from build123d import *

# Parameters (mm, degrees)
F0_W     = 50.8
F0_H     = 450.85
F0_R     = 3.770313
F1_DEPTH = 12.7
F2_R     = 4.167188
F3_DEPTH = 25.4
F5_DEPTH = 6.35


with BuildPart() as f1:
    # F0 (on Top) → F1 (new body)
    with BuildSketch(Plane.XY):
        Rectangle(F0_W, F0_H)
        with Locations((-17.5, -215.425)):
            Circle(F0_R, mode=Mode.SUBTRACT)
        with Locations((-17.5, -180.425)):
            Circle(F0_R, mode=Mode.SUBTRACT)
        with Locations((17.5, -215.425)):
            Circle(F0_R, mode=Mode.SUBTRACT)
        with Locations((17.5, -180.425)):
            Circle(F0_R, mode=Mode.SUBTRACT)
        with Locations((-17.5, 180.425)):
            Circle(F0_R, mode=Mode.SUBTRACT)
        with Locations((-17.5, 215.425)):
            Circle(F0_R, mode=Mode.SUBTRACT)
        with Locations((17.5, 180.425)):
            Circle(F0_R, mode=Mode.SUBTRACT)
        with Locations((17.5, 215.425)):
            Circle(F0_R, mode=Mode.SUBTRACT)
    extrude(amount=F1_DEPTH)

    # F2 (on face) → F3 (cut)
    with BuildSketch(Plane.XY.offset(12.7)):
        with Locations((-12.7, 0)):
            Circle(F2_R)
        with Locations((12.7, 0)):
            Circle(F2_R)
    extrude(amount=-F3_DEPTH, mode=Mode.SUBTRACT)

    # F4 (on face) → F5 (cut)
    with BuildSketch(Plane.XY.offset(12.7)):
        with BuildLine():
            ThreePointArc((-4.490128, -202.415128), (2.43004, -203.791635), (6.35, -197.925))
            ThreePointArc((6.35, -197.925), (5.866635, -195.49496), (4.490128, -193.434872))
            Line((4.490128, -193.434872), (-4.490128, -202.415128))
        make_face()
        with BuildLine():
            Line((-4.490128, -202.415128), (4.490128, -193.434872))
            ThreePointArc((4.490128, -193.434872), (-4.490128, -193.434872), (-4.490128, -202.415128))
        make_face()
    extrude(amount=-F5_DEPTH, mode=Mode.SUBTRACT)


solid = f1.part
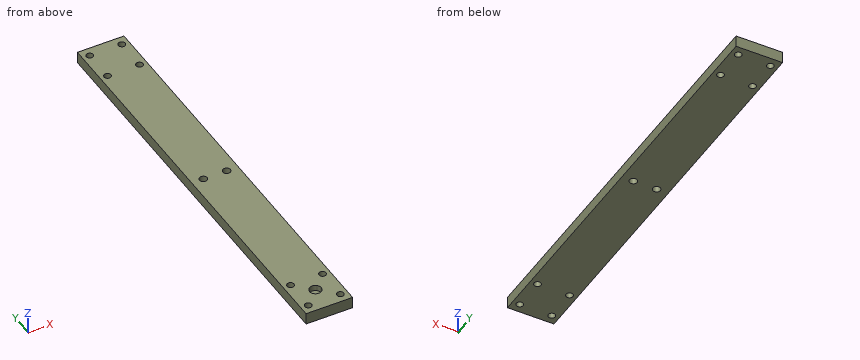
Check sheet for the modelled part. Datum: model origin and axes. Units: mm. Round coordinates to 2 decimals unless told otherwise and drop trailing zeros. Loops run counter-clockwise (first coordinate to the right, second up) from the corner with the lowest first, then second, coordinate; pieces in that order, holes last.
1. Scan lines: probe 1 along Y at (x, z) = (17.5, 4.75) (3 decimals); probe 2 along Y at (x, z) = (1, 11.75) (3 decimals); probe 3 along Y at (x, z) = (15, 10) (3 decimals). Record each from-to range of solid material in increasing order.
2. Gauge pin test, flat end, axial feed: pin 1 Ø4 at (x, y) = (-1.5, -196) entering from +Z. Record the tip position at first contact, or that the pin passes through.
3. Sectioned sample at B-B on z = 10.75. Give the number of separate pieces and of enclosed holes in the cut face, and give its area (3 significant figures).
4. Sectioned sample at A-A on y = 0. Record the boundary of the cut face in (x, z), and give its area (3 significant figures).
Recorded:
1. probe 1: y = -225.425 to -219.195, -211.655 to -184.195, -176.655 to 176.655, 184.195 to 211.655, 219.195 to 225.425
1. probe 2: y = -225.425 to -204.196, -191.654 to 225.425
1. probe 3: y = -225.425 to -218.247, -212.603 to -183.247, -177.603 to -3.475, 3.475 to 177.603, 183.247 to 212.603, 218.247 to 225.425
2. pin 1: stops at z = 6.35
3. separate pieces: 1
3. enclosed holes: 11
3. area: 22,300 mm2
4. outline: (-25.4, 0) - (-16.87, 0) - (-16.87, 12.7) - (-25.4, 12.7) - close; (-8.53, 0) - (8.53, 0) - (8.53, 12.7) - (-8.53, 12.7) - close; (16.87, 0) - (25.4, 0) - (25.4, 12.7) - (16.87, 12.7) - close
4. area: 433 mm2
